Autodesk Inventor part; units mm, degrees
ref_plane "YZ Plane" through (0, 0, 0) normal (1, 0, 0) x (0, 1, 0)
ref_plane "XZ Plane" through (0, 0, 0) normal (0, 1, 0) x (-1, 0, 0)
ref_plane "XY Plane" through (0, 0, 0) normal (0, 0, 1) x (1, 0, 0)
sketch "Sketch1" plane through (0, 0, 0) normal (0, 0, 1) x (1, 0, 0)
  circle A0 centre (0, 0) radius 6.35
  line L0 (7.3323, -0.0033) -> (3.6633, -6.3517)
  line L1 (3.6633, -6.3517) -> (-3.6691, -6.3483)
  line L2 (-3.6691, -6.3483) -> (-7.3323, 0.0033)
  line L3 (-7.3323, 0.0033) -> (-3.6633, 6.3517)
  line L4 (-3.6633, 6.3517) -> (3.6691, 6.3483)
  line L5 (3.6691, 6.3483) -> (7.3323, -0.0033)
  point P0 (5.5007, 3.1725)
  dimension "d0" = 12.7
extrude "Extrusion1" add sketch "Sketch1" along normal blind 749.3
properties part number "4-bar intake shaft (29.5)"
The listing builds one solid part. Answer for the finished solid, in the listing's coordinates (mm). Round coordinates to 2 decimals unless told otherwise and drop trailing zeros. Order: outer loops, then holes, each group sorted by start corner. A loop starts at its lowest first (then second) coordinate and runs counter-clockwise, first axis right, second up. Notation, with made-up numbers: (15.25, 39.25) -> (29.25, 39.25) arc R23 ccw to (29.25, 75.25) -> close; hole circle Ø4 at (15.5, 16). An arc over 180 degrees is marked (long way). Write each question's results on one line, items separated by ' | '. Start each with the question number.
Q1. This flat-tipped pin is pushed along its axis until it touches: pin 1 (3 mm diameter, centred on x = -5.5, z = 382.5, fed in from -Y). Where does it stop, or does it pass through?
Q2. Find section B-B (y = 2). Determine the outline of the cut face in (x, z), then the cut area to 3 significant figures.
Q3. Straight lines are drawn through the part: probe 1 along Y at (x, z) = (5.25, 62); probe 2 along Y at (x, z) = (2.25, 557); probe 3 along X at (y, z) = (0.25, 79.5). For each, find the intervals that lie inside material, in ascending order. Write a range as from..to.
Q4. Find section A-A (z = 231.5). Determine the outline of the cut face in (x, y).
Worked answers:
1) pin 1: stops at y = -5.77
2) outline: (-6.18, 0) -> (6.18, 0) -> (6.18, 749.3) -> (-6.18, 749.3) -> close | area: 9,260 mm2
3) probe 1: y = -3.61..3.61 | probe 2: y = -6.35..6.35 | probe 3: x = -7.19..7.19
4) outline: (-7.33, 0) -> (-3.67, -6.35) -> (3.66, -6.35) -> (7.33, 0) -> (3.67, 6.35) -> (-3.66, 6.35) -> close
